Design review of the part built by this model. Coordinates are the model's own, in mm. A direction names the side the tool comes from. Round coordinates to 2 decimals unless told otherwise and drop trailing zeros. Order: outer loops, then holes, each group sorted by start corner. A loop starts at its lowest first (then second) coordinate and runs counter-clockwise, first axis right, second up. Notation, with made-up numbers: M 61,75.25 L 88,75.25 A27 cw 88,104.25 Z; hole C 36,87 d4. An arc over 180 degrees is marked long. Write item = value, one per line. Start each with the question number.
```python
from build123d import *

# Parameters (mm, degrees)
ESBO_O1_W             = 12.8
ESBO_O1_H             = 12.3
CHANFRO1_SIZE         = 1
CORTE_EXTRUS_O1_DEPTH = 49.262718531
ESBO_O3_R             = 4.15
CORTE_EXTRUS_O2_DEPTH = 49.262718531
CHANFRO2_SIZE         = 0.5


with BuildPart() as part:
    # Esboço1 → Revolução1 (revolve)
    with BuildSketch(Plane.XY, mode=Mode.PRIVATE) as revolu_o1_sk:
        with Locations((26.6, 6.15)):
            Rectangle(ESBO_O1_W, ESBO_O1_H)
    revolve(revolu_o1_sk.sketch.rotate(Axis((0, -47.977777778, 0), (0, 1, 0)), 90), axis=Axis((0, -47.977777778, 0), (0, 1, 0)))

    # Chanfro1
    chanfro1_edges = [part.edges().sort_by_distance(p)[0] for p in [
        (0, 0, 33),
        (0, 0, 20.2),
        (0, 12.3, 20.2),
        (0, 12.3, 33),
    ]]
    chamfer(chanfro1_edges, length=CHANFRO1_SIZE)

    # Esboço2 → Corte-extrusão1 (cut, through all)
    with BuildSketch(Plane(origin=(0, 12.3, 0), x_dir=(1, 0, 0), z_dir=(0, 1, 0))):
        with BuildLine():
            Line((20.918742494, 17.850944302), (10.058223509, 13.898038663))
            Line((10.058223509, 13.898038663), (17.065166299, 1.761657744))
            Line((17.065166299, 1.761657744), (25.918742494, 9.190690264))
            ThreePointArc((25.918742494, 9.190690264), (23.815698604, 13.75), (20.918742494, 17.850944302))
        make_face()
        with BuildLine():
            Line((-5, 27.041634566), (-7.00694279, 15.659696407))
            Line((-7.00694279, 15.659696407), (7.00694279, 15.659696407))
            Line((7.00694279, 15.659696407), (5, 27.041634566))
            ThreePointArc((5, 27.041634566), (0, 27.5), (-5, 27.041634566))
        make_face()
        with BuildLine():
            Line((25.918742494, -9.190690264), (17.065166299, -1.761657744))
            Line((17.065166299, -1.761657744), (10.058223509, -13.898038663))
            Line((10.058223509, -13.898038663), (20.918742494, -17.850944302))
            ThreePointArc((20.918742494, -17.850944302), (23.815698604, -13.75), (25.918742494, -9.190690264))
        make_face()
        with BuildLine():
            Line((5, -27.041634566), (7.00694279, -15.659696407))
            Line((7.00694279, -15.659696407), (-7.00694279, -15.659696407))
            Line((-7.00694279, -15.659696407), (-5, -27.041634566))
            ThreePointArc((-5, -27.041634566), (0, -27.5), (5, -27.041634566))
        make_face()
        with BuildLine():
            Line((-20.918742494, -17.850944302), (-10.058223509, -13.898038663))
            Line((-10.058223509, -13.898038663), (-17.065166299, -1.761657744))
            Line((-17.065166299, -1.761657744), (-25.918742494, -9.190690264))
            ThreePointArc((-25.918742494, -9.190690264), (-23.815698604, -13.75), (-20.918742494, -17.850944302))
        make_face()
        with BuildLine():
            Line((-25.918742494, 9.190690264), (-17.065166299, 1.761657744))
            Line((-17.065166299, 1.761657744), (-10.058223509, 13.898038663))
            Line((-10.058223509, 13.898038663), (-20.918742494, 17.850944302))
            ThreePointArc((-20.918742494, 17.850944302), (-23.815698604, 13.75), (-25.918742494, 9.190690264))
        make_face()
    extrude(amount=-CORTE_EXTRUS_O1_DEPTH, mode=Mode.SUBTRACT)

    # Esboço3 → Corte-extrusão2 (cut, through all)
    with BuildSketch(Plane(origin=(0, 12.3, 0), x_dir=(1, 0, 0), z_dir=(0, 1, 0))):
        with Locations(Location((-26.5, 0, 0), (0, 0, 270))):
            Circle(ESBO_O3_R)
        with Locations(Location((-13.25, 22.9496732, 0), (0, 0, 270))):
            Circle(ESBO_O3_R)
        with Locations(Location((13.25, 22.9496732, 0), (0, 0, 270))):
            Circle(ESBO_O3_R)
        with Locations(Location((26.5, 0, 0), (0, 0, 270))):
            Circle(ESBO_O3_R)
        with Locations(Location((13.25, -22.9496732, 0), (0, 0, 270))):
            Circle(ESBO_O3_R)
        with Locations(Location((-13.25, -22.9496732, 0), (0, 0, 270))):
            Circle(ESBO_O3_R)
    extrude(amount=-CORTE_EXTRUS_O2_DEPTH, mode=Mode.SUBTRACT)

    # Chanfro2
    chanfro2_edges = [part.edges().sort_by_distance(p)[0] for p in [
        (-26.5, 0, -4.15),
        (-26.5, 12.3, -4.15),
        (-13.25, 0, -27.0996732),
        (-13.25, 12.3, -27.0996732),
        (13.25, 0, -27.0996732),
        (13.25, 12.3, -27.0996732),
        (26.5, 0, -4.15),
        (26.5, 12.3, -4.15),
        (13.25, 0, 18.7996732),
        (13.25, 12.3, 18.7996732),
        (-13.25, 0, 18.7996732),
        (-13.25, 12.3, 18.7996732),
    ]]
    chamfer(chanfro2_edges, length=CHANFRO2_SIZE)


solid = part.part
```
(1) Consider section A-A, the plane x = 0. Write out the cut boundary in (y, z).
(2) Consider section B-B, the plane z = 0. State how many separate pieces and enclosed holes the cut face has, then the cut area to 3 significant figures.
(3) For line 1 along X through (y, z) = (9.5, 22.5); line 2 along X through (y, z) = (7.5, -24.5); line 3 along Z through (x, y) = (11, 3.5), list the stretches that pass through material, from the lowest coordinate up. Write a range as [from, to].
(4) Insertion check: pin 1 (3 mm diameter, centred on x = -19, y = 11, fed in from -Z); pin 2 (6 mm diameter, centred on y = 6, z = 8, fed in from -X); pin 3 (2 mm diameter, centred on x = -1.5, y = 4, fed in from +Z). Each pin has a flat end and moves straight along its axis. Give the tip position at first contact, or say it passes through.
(5) Draft analysis for pull direction X (two halves, no side actions). For faces 4 (the face through (-22.81, 6.24, 6.58)), 5 (the face through (-21.5, 0, -0.1)), 6 (the face through (-17.107, 6.236, -16.464)), state which applies: pulls with the +X half, pulls with the -X half, needs draft (parallel to the pull), parting line crosses it, or undercut.
(6) For faces 1 (the face through (-10.2, 11.7, -17.9)), 2 (the face through (10.149, 6.222, -17.465)), 3 (the face through (-10.355, 0.604, 17.804)), list the 3-axis set-ups (+Z, -Z, +X, -X, +Y, -Y) from which the entire face can be reached by the end or side of a thin tool; tool diameter is ignored.
Completed:
q1.outline = M 0,-32 L 1,-33 L 11.3,-33 L 12.3,-32 L 12.3,-27.5 L 0,-27.5 Z; M 0,27.5 L 12.3,27.5 L 12.3,32 L 11.3,33 L 1,33 L 0,32 Z
q2.separate_pieces = 4
q2.enclosed_holes = 0
q2.area = 106 mm2
q3.line_1 = [-24.14, -17.38], [-9.12, -5.8], [5.8, 9.12], [17.38, 24.14]
q3.line_2 = [-22.11, -17.1], [-9.4, -5.45], [5.45, 9.4], [17.1, 22.11]
q3.line_3 = [-31.11, -26.44], [-19.46, -16.94], [16.94, 19.46], [26.44, 31.11]
q4.pin_1 = -27.98
q4.pin_2 = -32.62
q4.pin_3 = 33
q5.face_4 = undercut
q5.face_5 = needs draft
q5.face_6 = undercut
q6.face_1 = +Y
q6.face_2 = +Y, -Y
q6.face_3 = -Y
